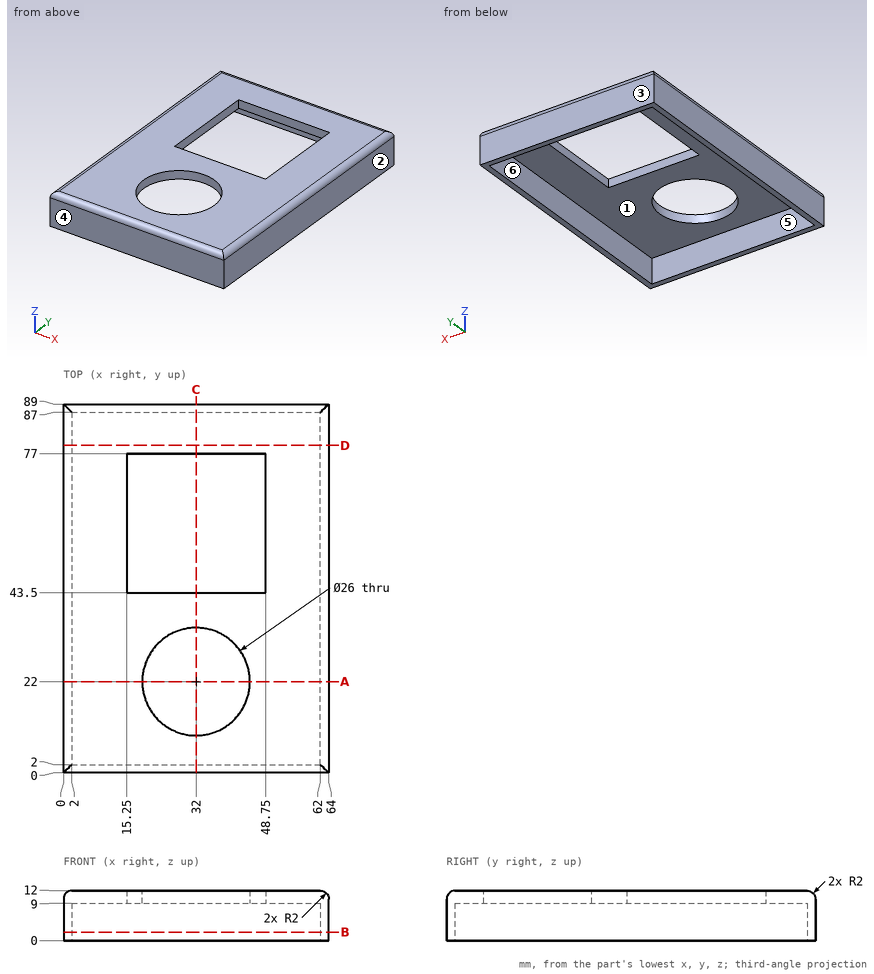
The drawing under review shows one solid part. Ordinate dimensions are in mm from its lowest x, y, z. A direction names the side the tool comes from. Round coordinates to 2 decimals unless told otherwise and drop trailing zeros. Loops run counter-clockwise (first coordinate to the right, second up) from the corner with the lowest first, then second, coordinate; pieces in that order, holes last. Notation, with made-up numbers: (-2.75, -25) -> (6.25, -25) arc R32 ccw to (6.25, 4) -> close; hole circle Ø11 at (13.5, 8.25). An arc over 180 degrees is marked (long way). Answer in a Markdown table with one row per item.
1) Consider section A-A, the plane y = 22. Write out the cut boundary in (x, z), plus the area to 3 significant figures.
Taken from the geometry:
| item | result |
|---|---|
| outline | (0, 0) -> (2, 0) -> (2, 9) -> (19, 9) -> (19, 12) -> (2, 12) arc R2 ccw to (0, 10) -> close; (45, 9) -> (62, 9) -> (62, 0) -> (64, 0) -> (64, 10) arc R2 ccw to (62, 12) -> (45, 12) -> close |
| area | 148 mm² |
2) Consider section B-B, the plane z = 2. Write out the cut boundary in (x, y), plus the area to 3 significant figures.
Taken from the geometry:
| item | result |
|---|---|
| outline | (0, 0) -> (64, 0) -> (64, 89) -> (0, 89) -> close; hole (2, 2) -> (62, 2) -> (62, 87) -> (2, 87) -> close |
| area | 596 mm² |
3) Consider section D-D, the plane y = 79. Write out the cut boundary in (x, z), plus the area to 3 significant figures.
Taken from the geometry:
| item | result |
|---|---|
| outline | (0, 0) -> (2, 0) -> (2, 9) -> (62, 9) -> (62, 0) -> (64, 0) -> (64, 10) arc R2 ccw to (62, 12) -> (2, 12) arc R2 ccw to (0, 10) -> close |
| area | 226 mm² |
4) Draft analysis for pull direction Y (two halves, no side actions). For the marked faces 3, 4, 5 and 6, state which applies: pulls with the +Y half, pulls with the -Y half, needs draft (parallel to the pull), parting line crosses it, or undercut.
Taken from the geometry:
| item | result |
|---|---|
| face 3 | pulls with the +Y half |
| face 4 | pulls with the -Y half |
| face 5 | undercut |
| face 6 | undercut |
5) Tool access review of the marked faces 1 and 2: name each direction out of +Z, -Z, +X, -X, +Y, -Y from which nothing blocks a thin tool from reaching the whole face with its end or side.
Taken from the geometry:
| item | result |
|---|---|
| face 1 | -Z |
| face 2 | +Z, -Z, +X, +Y, -Y |
6) Consider section C-C, the plane x = 32. Write out the cut boundary in (y, z), plus the area to 3 significant figures.
Taken from the geometry:
| item | result |
|---|---|
| outline | (0, 0) -> (2, 0) -> (2, 9) -> (9, 9) -> (9, 12) -> (2, 12) arc R2 ccw to (0, 10) -> close; (35, 9) -> (43.5, 9) -> (43.5, 12) -> (35, 12) -> close; (77, 9) -> (87, 9) -> (87, 0) -> (89, 0) -> (89, 10) arc R2 ccw to (87, 12) -> (77, 12) -> close |
| area | 123 mm² |
7) For pin 1 Ø18 at (x, y) = (27, 55) entering from -Z; pin 2 Ø2 at (x, y) = (55.5, 50) entering from -Z; pin 3 Ø0.9 at (y, z) = (58, 11) entering from -X, all flat-tipped, find the tip position at first contact; note any pin that passes through.
Taken from the geometry:
| item | result |
|---|---|
| pin 1 | passes through |
| pin 2 | stops at z = 9 |
| pin 3 | stops at x = 0.08 |
8) Wall thickness on line 1 along Y through (x, z) = (32, 9.8); line 2 along Y through (x, z) = (25, 3); line 3 along Y through (x, z) = (37.5, 10): over which ranges is each line inside the solid? List them lowest first.
Taken from the geometry:
| item | result |
|---|---|
| line 1 | y = 0 to 9, 35 to 43.5, 77 to 89 |
| line 2 | y = 0 to 2, 87 to 89 |
| line 3 | y = 0 to 10.22, 33.78 to 43.5, 77 to 89 |
